from build123d import *

# Parameters (mm, degrees)
SKETCH_W        = 36
SKETCH_H        = 10
PAD_DEPTH       = 15
SKETCH004_R     = 12.7
POCKET_DEPTH    = 10.001
CHAMFER_SIZE    = 0.5
SKETCH005_R     = 1.8
POCKET001_DEPTH = 15.001
FILLET_R        = 1


with BuildPart() as part:
    # Sketch → Pad (new body)
    with BuildSketch(Plane.XY):
        Rectangle(SKETCH_W, SKETCH_H)
    extrude(amount=PAD_DEPTH)

    # Sketch004 → Pocket (cut, through all)
    with BuildSketch(Plane(origin=(0, 5, 0), x_dir=(-1, 0, 0), z_dir=(0, 1, 0))):
        with Locations((0, 16)):
            Circle(SKETCH004_R)
    extrude(amount=-POCKET_DEPTH, mode=Mode.SUBTRACT)

    # Chamfer
    chamfer_edges = [part.edges().sort_by_distance(p)[0] for p in [
        (0, 5, 0),
        (18, 0, 0),
        (0, -5, 0),
        (-18, 0, 0),
    ]]
    chamfer(chamfer_edges, length=CHAMFER_SIZE)

    # Sketch005 → Pocket001 (cut, through all)
    with BuildSketch(Plane(origin=(0, 0, 0), x_dir=(1, 0, 0), z_dir=(0, 0, -1))):
        with Locations((15.160569, 0.454356)):
            Circle(SKETCH005_R)
        with Locations((-15.160569, 0.454356)):
            Circle(SKETCH005_R)
    extrude(amount=-POCKET001_DEPTH, mode=Mode.SUBTRACT)

    # Fillet
    fillet_edges = [part.edges().sort_by_distance(p)[0] for p in [
        (-18, -5, 7.75),
        (18, -5, 7.75),
        (18, 5, 7.75),
        (-18, 5, 7.75),
    ]]
    fillet(fillet_edges, radius=FILLET_R)


solid = part.part
Part model, mm, in its own coordinate system. Coordinates: 2 decimals unless noted, no trailing zeros. Order: outer loops, then holes, each group sorted by start corner. A loop starts at its lowest first (then second) coordinate and runs counter-clockwise, first axis right, second up. Notation, with made-up numbers: M 12.25,73 L 33.25,73 A23 ccw 33.25,83 Z; hole C -20.5,7 d1. An arc over 180 degrees is marked long. Use a Markdown table: item, result.
(1) Cut at C-C on z = 9. Write the cut outline in (x, y), then the cut area to 3 significant figures.
A:
| item | result |
|---|---|
| outline | M -18,-4 A1 ccw -17,-5 L -10.6,-5 L -10.6,5 L -17,5 A1 ccw -18,4 Z; M 10.6,-5 L 17,-5 A1 ccw 18,-4 L 18,4 A1 ccw 17,5 L 10.6,5 Z; hole C -15.16,-0.45 d3.6; hole C 15.16,-0.45 d3.6 |
| area | 127 mm^2 |
(2) Pull direction Y, two halves, no side cores. Call faces 1 (the cylindrical face through (15.991, 1.143, 7.395)), 2 (the cylindrical face through (17.699, 4.715, 7.707)), 3 (the flat face through (16.5, 1.2, 15)): released by +Y, released by -Y, zero draft, split by the parting line, or undercut.
A:
| item | result |
|---|---|
| face 1 | undercut |
| face 2 | released by +Y |
| face 3 | zero draft |
(3) Cut at D-D on x = -2.5. Write the cut outline in (y, z), then the cut area to 3 significant figures.
A:
| item | result |
|---|---|
| outline | M -5,0.5 L -4.5,0 L 4.5,0 L 5,0.5 L 5,3.55 L -5,3.55 Z |
| area | 35.2 mm^2 |
(4) Cut at B-B on y = 0.75. Write the cut outline in (x, z).
A:
| item | result |
|---|---|
| outline | M -18,0.5 L -17.5,0 L -16.5,0 L -16.5,15 L -18,15 Z; M -13.82,0 L 13.82,0 L 13.82,15 L 12.66,15 A12.7 cw -12.66,15 L -13.82,15 Z; M 16.5,0 L 17.5,0 L 18,0.5 L 18,15 L 16.5,15 Z |
(5) Probe L1, parallel to X at y = -1.5, z = 12.5; L2, parallel to X at y = 0.75, z = 2; L3, parallel to Y at x = -15, z = 3.5. List the from-to ranges inside material, lowest first.
A:
| item | result |
|---|---|
| L1 | x = -18 to -16.63, -13.7 to -12.21, 12.21 to 13.7, 16.63 to 18 |
| L2 | x = -18 to -16.5, -13.82 to 13.82, 16.5 to 18 |
| L3 | y = -5 to -2.25, 1.34 to 5 |
(6) Cut at A-A on z = 10.75. Write the cut outline in (x, y), then the cut area to 3 significant figures.
A:
| item | result |
|---|---|
| outline | M -18,-4 A1 ccw -17,-5 L -11.56,-5 L -11.56,5 L -17,5 A1 ccw -18,4 Z; M 11.56,-5 L 17,-5 A1 ccw 18,-4 L 18,4 A1 ccw 17,5 L 11.56,5 Z; hole C -15.16,-0.45 d3.6; hole C 15.16,-0.45 d3.6 |
| area | 108 mm^2 |
